Source: three-view drawing plus pictorial views. Frame: mm from the lowest corner of the part. Coordinates: 2 decimals unless noted, no trailing zeros. Write each loop counter-clockwise with the first axis right and the second up, starting at its lowest first coordinate (ties: lowest second). Pieces come first, ordered by that corner, then holes. Notation, with made-up numbers: (35.25, 81) - (43.25, 81) arc R25 ccw to (43.25, 97) - close; hole circle Ø5 at (-24.75, 31.25). An arc over 180 degrees is marked (long way). One line per item, written item: value.
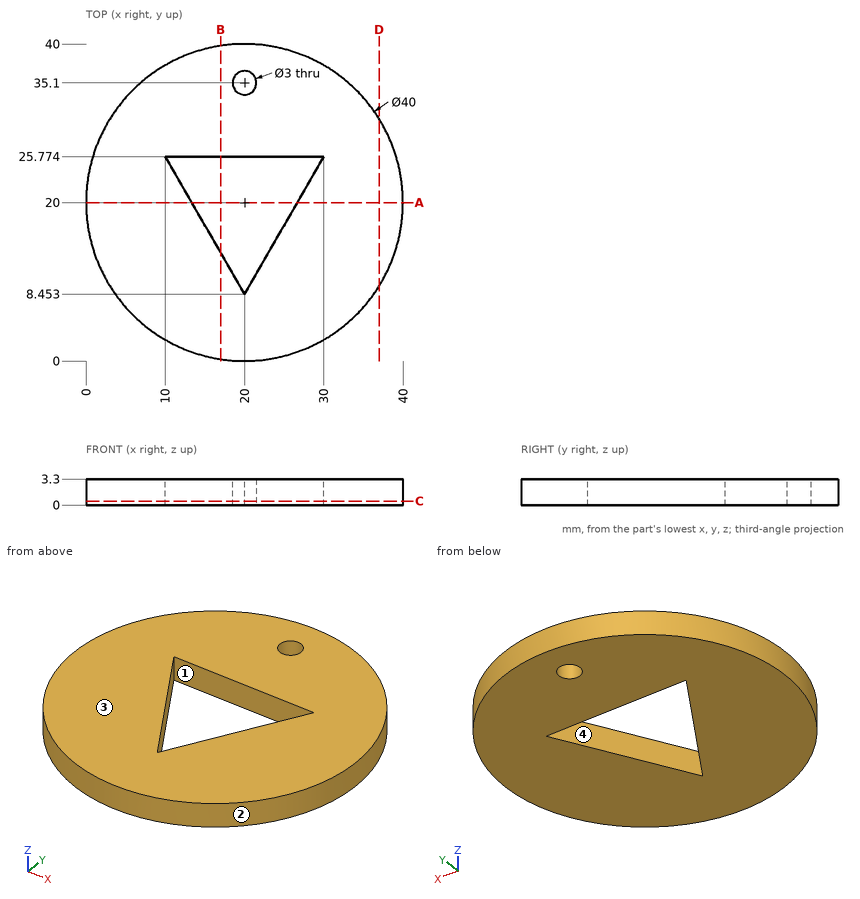
1) Material intervals for line 1 (Y direction, x = 21, z = 2.15) (1 decimal); line 2 (X direction, y = 23.5, z = 2.15); line 3 (Y direction, x = 18, z = 2.8) (1 decimal), sorted ascending.
Values found:
line 1: 0 to 10.2, 25.8 to 34, 36.2 to 40
line 2: 0.31 to 11.31, 28.69 to 39.69
line 3: 0.1 to 11.9, 25.8 to 39.9
2) Contact query for flat-ended pins moving along their axis: P1, Ø5, axis at x = 12, y = 20, coming from the -Z side; P2, Ø1.5, axis at y = 25, z = 1.5, coming from the -X side; P3, Ø1.6, axis at x = 21, z = 1.5, coming from the -Y side; P4, Ø1.5, axis at x = 16, z = 1, coming from the -Y side. Output: stop coordinate, or through.
Values found:
P1: z = 0
P2: x = 0.46
P3: y = 0
P4: y = 0.27
3) Draft query along X for the marked faces 1, 2, 3 and 4. Return one class per face: released by +X, released by -X, zero draft, split by the parting line, or undercut.
Values found:
face 1: undercut
face 2: split by the parting line
face 3: zero draft
face 4: undercut
4) Section query B-B on x = 17. Output: boundary loops of the cut face in (y, z).
Values found:
outline: (0.23, 0) - (13.65, 0) - (13.65, 3.3) - (0.23, 3.3) - close; (25.77, 0) - (39.77, 0) - (39.77, 3.3) - (25.77, 3.3) - close
5) Section query A-A on y = 20. Output: boundary loops of the cut face in (x, z).
Values found:
outline: (0, 0) - (13.33, 0) - (13.33, 3.3) - (0, 3.3) - close; (26.67, 0) - (40, 0) - (40, 3.3) - (26.67, 3.3) - close
6) Section query D-D on x = 37. Output: boundary loops of the cut face in (y, z) (1 decimal).
Values found:
outline: (9.5, 0) - (30.5, 0) - (30.5, 3.3) - (9.5, 3.3) - close
7) Section query C-C on z = 0.5. Output: boundary loops of the cut face in (x, y), then the cut area to 3 significant figures.
Values found:
outline: circle Ø40 at (20, 20); hole (10, 25.77) - (20, 8.45) - (30, 25.77) - close; hole circle Ø3 at (20, 35.1)
area: 1,080 mm2
